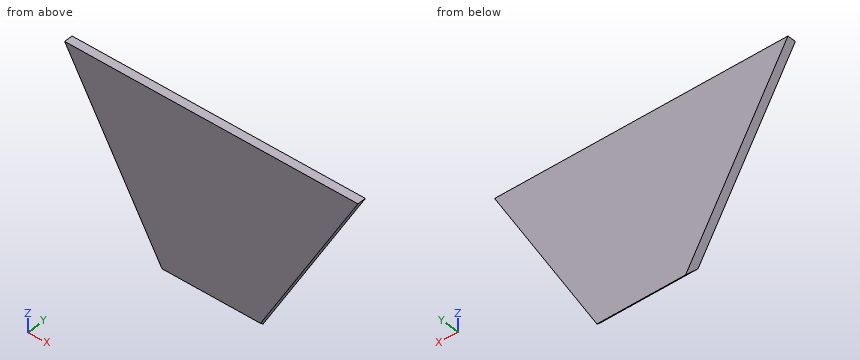
from build123d import *

# Parameters (mm, degrees)
BOSS_EXTRUDE1_DEPTH            = 6.35
CUT_EXTRUDE1_REACH             = 111.22
CUT_EXTRUDE1_DIRECTION_2_REACH = 111.22


with BuildPart() as part:
    # Sketch2 → Boss-Extrude1 (new body)
    with BuildSketch(Plane(origin=(0, 0, 0), x_dir=(1, 0, 0), z_dir=(0, 1, 0))):
        Polygon((-109.22, -85.086141102), (-33.02, 46.896130435), (33.02, 46.896130435), (109.22, -85.086141102), align=None)
    extrude(amount=BOSS_EXTRUDE1_DEPTH)

    # Sketch4 → Cut-Extrude1 (cut, up to next)
    with BuildSketch(Plane(origin=(0, 0, 0), x_dir=(0, 0, -1), z_dir=(1, 0, 0)), mode=Mode.PRIVATE) as cut_extrude1_sk1:
        Polygon((46.896130435, 6.35), (40.546130435, 0), (46.896130435, 0), align=None)
    cut_extrude1_tool1 = extrude(cut_extrude1_sk1.sketch, amount=-CUT_EXTRUDE1_REACH, mode=Mode.PRIVATE) & part.part
    add(cut_extrude1_tool1.solids().sort_by_distance((0, 2.116667, -44.779464))[0], mode=Mode.SUBTRACT)

    # Sketch4 → Cut-Extrude1 direction 2 (cut, up to next)
    with BuildSketch(Plane(origin=(0, 0, 0), x_dir=(0, 0, -1), z_dir=(1, 0, 0)), mode=Mode.PRIVATE) as cut_extrude1_direction_2_sk1:
        Polygon((46.896130435, 6.35), (40.546130435, 0), (46.896130435, 0), align=None)
    cut_extrude1_direction_2_tool1 = extrude(cut_extrude1_direction_2_sk1.sketch, amount=CUT_EXTRUDE1_DIRECTION_2_REACH, mode=Mode.PRIVATE) & part.part
    add(cut_extrude1_direction_2_tool1.solids().sort_by_distance((0, 2.116667, -44.779464))[0], mode=Mode.SUBTRACT)


solid = part.part
Input: part model. Units: mm. Frame: model coordinates. Round coordinates to 2 decimals unless told otherwise and drop trailing zeros. Order: outer loops, then holes, each group sorted by start corner. A loop starts at its lowest first (then second) coordinate and runs counter-clockwise, first axis right, second up. Notation, with made-up numbers: (79.25, 84.25) - (137.25, 84.25) arc R19 ccw to (137.25, 99.25) - close; hole circle Ø9 at (9.5, 28). An arc over 180 degrees is marked (long way). Use a Markdown table: item, result.
1. First-contact query: pin 1 (3 mm diameter, centred on y = 4, z = 49.5, fed in from -X); pin 2 (10 mm diameter, centred on x = 65, z = 17, fed in from -Y); pin 3 (3 mm diameter, centred on y = 4, z = -11.5, fed in from -X); pin 4 (1.5 mm diameter, centred on x = 50.5, y = 5, fed in from -Z). Flat tips, straight axial feed; report the tip coordinate or a pass-through.
Evaluation:
| item | result |
|---|---|
| pin 1 | x = -89.54 |
| pin 2 | y = 0 |
| pin 3 | x = -54.32 |
| pin 4 | z = -17.92 |
2. Section A-A on x = -18. Return the cut outline in (y, z), then the cut area to 3 significant figures.
Evaluation:
| item | result |
|---|---|
| outline | (0, -40.55) - (6.35, -46.9) - (6.35, 85.09) - (0, 85.09) - close |
| area | 818 mm^2 |
3. Material intervals for probe 1 along Z at (x, y) = (-57.5, 3); probe 2 along X at (y, z) = (4, 26.5); probe 3 along X at (y, z) = (4, -4.5), sorted ascending.
Evaluation:
| item | result |
|---|---|
| probe 1 | -4.5 to 85.09 |
| probe 2 | -75.4 to 75.4 |
| probe 3 | -57.5 to 57.5 |
4. Section B-B on z = -34.5. Return the cut outline in (x, y).
Evaluation:
| item | result |
|---|---|
| outline | (-40.18, 0) - (40.18, 0) - (40.18, 6.35) - (-40.18, 6.35) - close |
